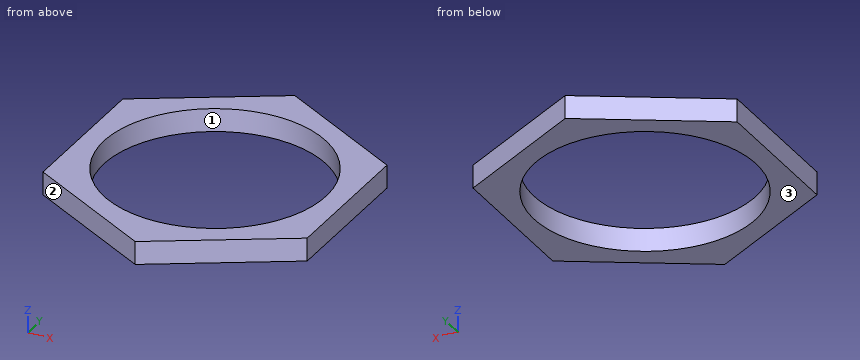
Autodesk Inventor part; units mm, degrees
ref_plane "YZ Plane" through (0, 0, 0) normal (1, 0, 0) x (0, 1, 0)
ref_plane "XZ Plane" through (0, 0, 0) normal (0, 1, 0) x (-1, 0, 0)
ref_plane "XY Plane" through (0, 0, 0) normal (0, 0, 1) x (1, 0, 0)
sketch "Sketch1" plane through (0, 0, 0) normal (0, 0, 1) x (1, 0, 0)
  line L0 (0, 16.5122) -> (14.3, 8.2561)
  line L1 (14.3, 8.2561) -> (14.3, -8.2561)
  line L2 (14.3, -8.2561) -> (0, -16.5122)
  line L3 (0, -16.5122) -> (-14.3, -8.2561)
  line L4 (-14.3, -8.2561) -> (-14.3, 8.2561)
  line L5 (-14.3, 8.2561) -> (0, 16.5122)
  point P0 (0, 0)
  point P1 (0, 0)
  dimension "d0" = 28.6
extrude "Extrusion1" add sketch "Sketch1" along normal blind 2.5
sketch "Sketch2" plane through (0, 0, 2.5) normal (0, 0, 1) x (1, 0, 0)
  point P0 (0, 0)
hole "Hole1" at (0, 0, 2.5) direction (0, 0, -1) diameter 24.0284 end through all
properties part number "USB NUT"
The listing builds one solid part. Answer for the finished solid, in the listing's coordinates (mm). Face numbers are marked on the shaded views. Round coordinates to 2 decimals unless told otherwise and drop trailing zeros. Loops run counter-clockwise (first coordinate to the right, second up) from the corner with the lowest first, then second, coordinate; pieces in that order, holes last. Notation, with made-up numbers: M -10,83.5 L 6,83.5 A15 ccw 6,107.5 Z; hole C 69.5,24.25 d4. An arc over 180 degrees is marked long. Return JSON: item names as keys, results as strings.
Q1. Find section D-D, the plane y = 14. Determine the outline of the cut face in (x, z), plus the area to 3 significant figures.
Results list:
{"outline": "M -4.35,0 L 4.35,0 L 4.35,2.5 L -4.35,2.5 Z", "area": "21.8 mm2"}
Q2. Find section B-B, the plane z = 2.05. Determine the outline of the cut face in (x, y), plus the area to 3 significant figures.
Results list:
{"outline": "M -14.3,-8.26 L 0,-16.51 L 14.3,-8.26 L 14.3,8.26 L 0,16.51 L -14.3,8.26 Z; hole C 0,0 d24.03", "area": "255 mm2"}
Q3. The mould has two halves that part along X. Classify the marked faces 1, 2 and 3: released by +X, released by -X, zero draft, split by the parting line, or undercut.
Results list:
{"face 1": "undercut", "face 2": "released by -X", "face 3": "zero draft"}
Q4. Find the intervals of material crossed by line 1 along Y through (x, z) = (0, 1.05); line 2 along X through (y, z) = (0, 0.65); line 3 along Y through (x, z) = (9, 1.85), in increasing order. Write a range as from..to.
Results list:
{"line 1": "y = -16.51..-12.01, 12.01..16.51", "line 2": "x = -14.3..-12.01, 12.01..14.3", "line 3": "y = -11.32..-7.96, 7.96..11.32"}
Q5. Find section C-C, the plane x = -8. Determine the outline of the cut face in (y, z), plus the area to 3 significant figures.
Results list:
{"outline": "M -11.89,0 L -8.96,0 L -8.96,2.5 L -11.89,2.5 Z; M 8.96,0 L 11.89,0 L 11.89,2.5 L 8.96,2.5 Z", "area": "14.7 mm2"}
Q6. Find section A-A, the plane y = 0. Determine the outline of the cut face in (x, z).
Results list:
{"outline": "M -14.3,0 L -12.01,0 L -12.01,2.5 L -14.3,2.5 Z; M 12.01,0 L 14.3,0 L 14.3,2.5 L 12.01,2.5 Z"}
